Autodesk Fusion 360 part; units mm, degrees
sketch "Sketch1" plane through (0, 0, 0) normal (0, 1, 0) x (1, 0, 0)
  line L0 (0, 0) -> (50, 0)
  line L1 (50, 0) -> (50, 30)
  line L2 (50, 30) -> (0, 30)
  line L3 (0, 30) -> (0, 0)
  line L4 (49, 29) -> (1, 29)
  line L5 (1, 29) -> (1, 1)
  line L6 (1, 1) -> (49, 1)
  line L7 (49, 1) -> (49, 29)
  dimension "d16" = 50
  dimension "d17" = 30
extrude "Extrude5" add sketch "Sketch1" along normal blind 30
extrude "Extrude6" add sketch "Sketch1" along normal blind 1 contours L4 L5 L6 L7
equation "thickness = 1 mm"
equation "depth = 30 mm"
equation "width = 50 mm"
equation "height = 30 mm"
equation "d16 = width"
equation "d17 = depth"
equation "d19 = height"
equation "d21 = thickness"
For this review, take the finished solid that the model builds, in its own axes (mm). A direction names the side the tool comes from. Coordinates: 2 decimals unless noted, no trailing zeros. Loops run counter-clockwise (first coordinate to the right, second up) from the corner with the lowest first, then second, coordinate; pieces in that order, holes last. Notation, with made-up numbers: (52, 52.25) - (79, 52.25) arc R24 cw to (79, 87.25) - close; hole circle Ø3 at (81, 15.25). An arc over 180 degrees is marked (long way). Return JSON: item names as keys, results as strings.
Item 1: For faces 5 (the flat face through (25, 15, 0)), 6 (the flat face through (49, 15, -15)), list the 3-axis set-ups (+Z, -Z, +X, -X, +Y, -Y) from which the entire face can be reached by the end or side of a thin tool; tool diameter is ignored.
Determined:
{"face 5": "+Z, +X, -X, +Y, -Y", "face 6": "+Y"}
Item 2: Insertion check: pin 1 (5 mm diameter, centred on x = 25.5, z = -14.5, fed in from +Y). The pin has a flat end and moves straight along its axis. Give the tip position at first contact, or say it passes through.
Determined:
{"pin 1": "stops at y = 1"}
Item 3: Mouldability with a two-part tool opening along Z and no side actions: class faces 1 (the flat face through (25, 15, -30)), 2 (the flat face through (25, 15, -1)), 3 (the flat face through (25, 1, -15)), 4 (the flat face through (25, 0, -15)) as pulls with the +Z half, pulls with the -Z half, needs draft (parallel to the pull), parting line crosses it, or undercut.
Determined:
{"face 1": "pulls with the -Z half", "face 2": "undercut", "face 3": "undercut", "face 4": "needs draft"}
Item 4: For line 1 (X direction, y = 10.75, z = -7.75); line 2 (Z direction, x = 44, y = 7.75); line 3 (Y direction, x = 45, z = -11), list the stretches that pass through material, from the lowest coordinate up.
Determined:
{"line 1": "x = 0 to 1, 49 to 50", "line 2": "z = -30 to -29, -1 to 0", "line 3": "y = 0 to 1"}
Item 5: Take a section at B-B (z = -8.25). Give the boundary of the cut face in (x, y).
Determined:
{"outline": "(0, 0) - (50, 0) - (50, 30) - (49, 30) - (49, 1) - (1, 1) - (1, 30) - (0, 30) - close"}
Item 6: Take a section at A-A (y = 21.25). Give the boundary of the cut face in (x, z), then the cut area to 3 significant figures.
Determined:
{"outline": "(0, -30) - (50, -30) - (50, 0) - (0, 0) - close; hole (1, -29) - (49, -29) - (49, -1) - (1, -1) - close", "area": "156 mm2"}
Item 7: Take a section at C-C (x = 10). Give the boundary of the cut face in (y, z), then the cut area to 3 significant figures.
Determined:
{"outline": "(0, -30) - (30, -30) - (30, -29) - (1, -29) - (1, -1) - (30, -1) - (30, 0) - (0, 0) - close", "area": "88.0 mm2"}
